from build123d import *

# Parameters (mm, degrees)
SKETCH9_W  = 13.112773862
SKETCH9_H  = 9
SKETCH11_W = 12
SKETCH11_H = 8.89


with BuildPart() as part:
    # Sketch1 → Revolve2 (revolve)
    with BuildSketch(Plane.XY, mode=Mode.PRIVATE) as revolve2_sk:
        Polygon((52.912966218, 65), (-117.087033782, 65), (-113.087033782, 61), (48.912966218, 61), align=None)
    revolve(revolve2_sk.sketch.rotate(Axis((-117.087033782, 0, 0), (1, 0, 0)), 180), axis=Axis((-117.087033782, 0, 0), (1, 0, 0)))

    # Sketch9 → Revolve4 (revolve)
    with BuildSketch(Plane.XY, mode=Mode.PRIVATE) as revolve4_sk:
        with Locations((-87.162646851, 69.5)):
            Rectangle(SKETCH9_W, SKETCH9_H)
    revolve(revolve4_sk.sketch.rotate(Axis((-161.549470518, 0, 0), (1, 0, 0)), 180), axis=Axis((-161.549470518, 0, 0), (1, 0, 0)))

    # Sketch11 → Revolve5 (revolve)
    with BuildSketch(Plane.XY, mode=Mode.PRIVATE) as revolve5_sk:
        with Locations((23.544966218, 69.445)):
            Rectangle(SKETCH11_W, SKETCH11_H)
    revolve(revolve5_sk.sketch.rotate(Axis((-147.745174043, 0, 0), (1, 0, 0)), 180), axis=Axis((-147.745174043, 0, 0), (1, 0, 0)))


solid = part.part
Input: part model. Units: mm. Frame: model coordinates. A direction names the side the tool comes from. Coordinates: 2 decimals unless noted, no trailing zeros. Write each loop counter-clockwise with the first axis right and the second up, starting at its lowest first coordinate (ties: lowest second). Pieces come first, ordered by that corner, then holes. Notation, with made-up numbers: M 1,-35 L 12,-35 A22 cw 12,-14 Z; hole C 36,-35 d11. An arc over 180 degrees is marked long. Answer as a JSON object with one key per item and string values. Group by question number.
(1) Section C-C on x = -101. Output: boundary loops of the cut face in (y, z).
(2) Set-up query: faces 1 (the face through (-105.57, -62, -19.52)), 2 (the face through (-80.606, -0.3, 65.4)), 3 (the face through (29.545, -0.3, 65.3)), 4 (the face through (-30.95, 13.22, 59.55)). Return all of +Z, -Z, +X, -X, +Y, -Y with unobstructed straight access to the full face (end or side cutting, diameter ignored); none if empty.
(3) Ray query, line 1 along Z through (x, y) = (-43, 0); line 2 along Y through (x, z) = (25.5, 46); line 3 along X through (y, z) = (-67, 15.5). Return the intervals inside material, ascending. Write a range as [from, to].
(4) Section A-A on z = 0. Output: boundary loops of the cut face in (x, y), plus the area to 3 significant figures.
(5) Contact query for flat-ended pins moving along their axis: P1, Ø2, axis at x = 26.5, z = -57, coming from the +Y side; P2, Ø4, axis at x = 5, y = 1.5, coming from the -Z side; P3, Ø12, axis at x = -7.5, z = -43.5, coming from the -Y side; P4, Ø1.5, axis at y = -46.5, z = -36.5, coming from the -X side. Output: stop coordinate, or through.
(6) Mould query, pull axis X, two halves, no side actions, for faces 5 (the face through (-93.719, -0.3, 65.4)), 6 (the face through (-32.22, -62, -19.52)), 7 (the face through (17.545, -0.3, 65.3)), 8 (the face through (23.629, 16.018, 72.133)). Classes: pulls with the +X half, pulls with the -X half, needs draft (parallel to the pull), parting line crosses it, or undercut.
Result set:
{
 "1": {"outline": "C 0,0 d130; hole C 0,0 d122"},
 "2": {"face 1": "-X", "face 2": "none", "face 3": "+X", "face 4": "+X, -X"},
 "3": {"line 1": "z = [-65, -61], [61, 65]", "line 2": "y = [-57.83, -40.06], [40.06, 57.83]", "line 3": "x = [-93.72, -80.61], [17.54, 29.54]"},
 "4": {"outline": "M -117.09,-65 L -93.72,-65 L -93.72,-74 L -80.61,-74 L -80.61,-65 L 17.54,-65 L 17.54,-73.89 L 29.54,-73.89 L 29.54,-65 L 52.91,-65 L 48.91,-61 L -113.09,-61 Z; M -117.09,65 L -113.09,61 L 48.91,61 L 52.91,65 L 29.54,65 L 29.54,73.89 L 17.54,73.89 L 17.54,65 L -80.61,65 L -80.61,74 L -93.72,74 L -93.72,65 Z", "area": "1,780 mm2"},
 "5": {"P1": "stops at y = 48.21", "P2": "stops at z = -65", "P3": "stops at y = -53.09", "P4": "passes through"},
 "6": {"face 5": "pulls with the -X half", "face 6": "undercut", "face 7": "undercut", "face 8": "needs draft"}
}
